Input: part model. Units: mm. Frame: model coordinates. A direction names the side the tool comes from. Round coordinates to 2 decimals unless told otherwise and drop trailing zeros. Write each loop counter-clockwise with the first axis right and the second up, starting at its lowest first coordinate (ties: lowest second). Pieces come first, ordered by that corner, then holes. Notation, with made-up numbers: (31.5, -17.75) -> (45.5, -17.75) arc R21 ccw to (45.5, 3.25) -> close; hole circle Ø11 at (10.25, -31.5). An arc over 180 degrees is marked (long way). Write item = value, one per line. Start each with the question number.
```python
from build123d import *

# Parameters (mm, degrees)
SKETCH1_W               = 80
SKETCH1_H               = 45
BOSS_EXTRUDE1_DEPTH     = 80
SHELL1_T                = -3
CUT_EXTRUDE3_DEPTH      = 101.124921973
CUT_EXTRUDE3_DEPTH_BACK = 101.124921973
SKETCH1_3_R             = 2


with BuildPart() as part:
    # Sketch1 → Boss-Extrude1 (new body)
    with BuildSketch(Plane.XY):
        with Locations((0, 22.5)):
            Rectangle(SKETCH1_W, SKETCH1_H)
    extrude(amount=BOSS_EXTRUDE1_DEPTH)

    # Shell1
    shell1_openings = [part.faces().sort_by_distance(p)[0] for p in [
        (0, 45, 40),
    ]]
    offset(amount=SHELL1_T, openings=shell1_openings, kind=Kind.INTERSECTION)

    # Sketch1_3 → Cut-Extrude3 (cut, two sides: drawn at the far end of the back side and taken through both)
    with BuildSketch(Plane.XY.offset(-CUT_EXTRUDE3_DEPTH_BACK)):
        with Locations(Location((-35, 40, 0), (0, 0, 180))):
            Circle(SKETCH1_3_R)
        with Locations((35, 40)):
            Circle(SKETCH1_3_R)
    extrude(amount=CUT_EXTRUDE3_DEPTH + CUT_EXTRUDE3_DEPTH_BACK, mode=Mode.SUBTRACT)


solid = part.part
```
1. Section C-C (z = 12). Output: boundary loops of the cut face in (x, y), then the cut area to 3 significant figures.
2. Section A-A (x = 35). Output: boundary loops of the cut face in (y, z).
3. Section D-D (x = -2). Output: boundary loops of the cut face in (y, z), then the cut area to 3 significant figures.
4. Mould query, pull axis Z, two halves, no side actions, for faces 3 (the flat face through (-1, 23, 80)), 4 (the flat face through (-1, 24, 3)), 5 (the flat face through (40, 22, 39)). Classes: pulls with the +Z half, pulls with the -Z half, needs draft (parallel to the pull), parting line crosses it, or undercut.
5. Reachability of faces 1 (the cylindrical face through (35.923, 38.226, 1.479)), 2 (the flat face through (37, 24, 39)) from +Z, -Z, +X, -X, +Y, -Y: full face, straight path, thin tool, end or side. Return the list, or none.
6. Section B-B (y = 13). Output: boundary loops of the cut face in (x, z), then the cut area to 3 significant figures.
7. Line query: line 1 along Z through (x, y) = (1.5, 19); line 2 along Y through (x, z) = (35, 78.95); line 3 along X through (y, z) = (36.5, 16). Output: solid intervals per line, ascending.
8. Pin query (flat end, axial travel): P1, Ø3, axis at x = -35, y = 40, coming from the +Z side. Return the tip coordinate at first contact, or that it passes through.
Check sheet entries:
q1.outline = (-40, 0) -> (40, 0) -> (40, 45) -> (37, 45) -> (37, 3) -> (-37, 3) -> (-37, 45) -> (-40, 45) -> close
q1.area = 492 mm2
q2.outline = (0, 0) -> (38, 0) -> (38, 3) -> (3, 3) -> (3, 77) -> (38, 77) -> (38, 80) -> (0, 80) -> close; (42, 0) -> (45, 0) -> (45, 3) -> (42, 3) -> close; (42, 77) -> (45, 77) -> (45, 80) -> (42, 80) -> close
q3.outline = (0, 0) -> (45, 0) -> (45, 3) -> (3, 3) -> (3, 77) -> (45, 77) -> (45, 80) -> (0, 80) -> close
q3.area = 492 mm2
q4.face_3 = pulls with the +Z half
q4.face_4 = undercut
q4.face_5 = needs draft
q5.face_1 = +Z, -Z
q5.face_2 = +Y
q6.outline = (-40, 0) -> (40, 0) -> (40, 80) -> (-40, 80) -> close; hole (-37, 3) -> (37, 3) -> (37, 77) -> (-37, 77) -> close
q6.area = 924 mm2
q7.line_1 = 0 to 3, 77 to 80
q7.line_2 = 0 to 38, 42 to 45
q7.line_3 = -40 to -37, 37 to 40
q8.P1 = through
